Autodesk Inventor part; units mm, degrees
ref_plane "YZ Plane" through (0, 0, 0) normal (1, 0, 0) x (0, 1, 0)
ref_plane "XZ Plane" through (0, 0, 0) normal (0, 1, 0) x (-1, 0, 0)
ref_plane "XY Plane" through (0, 0, 0) normal (0, 0, 1) x (1, 0, 0)
sketch "Sketch1" plane through (0, 0, 0) normal (0, 1, 0) x (-1, 0, 0)
  line L0 (-152.4, 28.575) -> (152.4, 28.575)
  line L1 (152.4, 28.575) -> (152.4, -28.575)
  line L2 (152.4, -28.575) -> (-152.4, -28.575)
  line L3 (-152.4, -28.575) -> (-152.4, 28.575)
  line L4 (-152.4, 28.575) -> (152.4, -28.575) construction
  line L5 (152.4, 28.575) -> (-152.4, -28.575) construction
  point P0 (0, 0)
  dimension "d0" = 304.8
  dimension "d1" = 57.15
extrude "Extrusion1" add sketch "Sketch1" along normal blind 3.175
sketch "Sketch2" plane through (0, 3.175, 0) normal (0, 1, 0) x (1, 0, 0)
  line L0 (152.4, 28.575) -> (-152.4, 28.575)
  line L1 (-152.4, -28.575) -> (152.4, -28.575)
  line L2 (0, -15.875) -> (-152.4, -15.875)
  line L3 (-152.4, 28.575) -> (-152.4, -28.575)
  line L4 (0, -15.875) -> (152.4, -15.875)
  line L5 (0, 15.875) -> (-152.4, 15.875)
  line L6 (0, 15.875) -> (152.4, 15.875)
  line L7 (152.4, -28.575) -> (152.4, 28.575)
  line L8 (-152.4, -15.875) -> (-107.95, -15.875)
  line L9 (-107.95, -15.875) -> (-63.5, -15.875)
  line L10 (-63.5, -15.875) -> (-19.05, -15.875)
  line L11 (-19.05, -15.875) -> (25.4, -15.875)
  line L12 (25.4, -15.875) -> (69.85, -15.875)
  line L13 (69.85, -15.875) -> (114.3, -15.875)
  line L14 (-152.4, 15.875) -> (-127, 15.875)
  line L15 (-127, 15.875) -> (-50.8, 15.875)
  line L16 (-50.8, 15.875) -> (25.4, 15.875)
  line L17 (25.4, 15.875) -> (101.6, 15.875)
  point P0 (0, 0)
  dimension "d8" = 44.45
  dimension "d9" = 44.45
  dimension "d10" = 44.45
  dimension "d11" = 44.45
  dimension "d12" = 44.45
  dimension "d13" = 44.45
  dimension "d14" = 25.4
  dimension "d15" = 76.2
  dimension "d16" = 76.2
  dimension "d17" = 76.2
hole "Hole1" at (-107.95, 3.175, 15.875) at (-63.5, 3.175, 15.875) at (-19.05, 3.175, 15.875) at (25.4, 3.175, 15.875) at (69.85, 3.175, 15.875) at (114.3, 3.175, 15.875) direction (0, -1, 0) diameter 5.1054 end through all
sketch "Sketch3" plane through (0, 3.175, 0) normal (0, 1, 0) x (1, 0, 0)
  line L0 (152.4, 28.575) -> (-152.4, 28.575)
  line L1 (-152.4, -28.575) -> (152.4, -28.575)
  line L2 (0, -15.875) -> (-152.4, -15.875)
  line L3 (-152.4, 28.575) -> (-152.4, -28.575)
  line L4 (0, -15.875) -> (152.4, -15.875)
  line L5 (0, 15.875) -> (-152.4, 15.875)
  line L6 (0, 15.875) -> (152.4, 15.875)
  line L7 (152.4, -28.575) -> (152.4, 28.575)
  line L8 (-152.4, -15.875) -> (-107.95, -15.875)
  line L9 (-107.95, -15.875) -> (-63.5, -15.875)
  line L10 (-63.5, -15.875) -> (-19.05, -15.875)
  line L11 (-19.05, -15.875) -> (25.4, -15.875)
  line L12 (25.4, -15.875) -> (69.85, -15.875)
  line L13 (69.85, -15.875) -> (114.3, -15.875)
  line L14 (-152.4, 15.875) -> (-127, 15.875)
  line L15 (-127, 15.875) -> (-50.8, 15.875)
  line L16 (-50.8, 15.875) -> (25.4, 15.875)
  line L17 (25.4, 15.875) -> (101.6, 15.875)
  point P0 (0, 0)
  point P1 (0, 0)
  dimension "d25" = 44.45
  dimension "d26" = 44.45
  dimension "d27" = 44.45
  dimension "d28" = 44.45
  dimension "d29" = 44.45
  dimension "d30" = 44.45
  dimension "d31" = 25.4
  dimension "d32" = 76.2
  dimension "d33" = 76.2
  dimension "d34" = 76.2
hole "Hole2" at (-127, 3.175, -15.875) at (-50.8, 3.175, -15.875) at (25.4, 3.175, -15.875) at (101.6, 3.175, -15.875) direction (0, -1, 0) diameter 3.81 end through all
properties part number "Rack-Elondo-Bracket"
Check sheet for the modelled part. Datum: model origin and axes. Units: mm. Round coordinates to 2 decimals unless told otherwise and drop trailing zeros. Loops run counter-clockwise (first coordinate to the right, second up) from the corner with the lowest first, then second, coordinate; pieces in that order, holes last. Notation, with made-up numbers: (18.25, -20) - (72.25, -20) arc R30 cw to (72.25, 18) - close; hole circle Ø8 at (20, 6.25). An arc over 180 degrees is marked (long way). Write item = value, one per line. Start each with the question number.
Q1. Release check for a two-part mould opening along Z. For faces 1 (the face through (2, 0, 0)), 2 (the face through (67.32, 1.57, 15.54)) record: pulls with the +Z half, pulls with the -Z half, needs draft (parallel to the pull), parting line crosses it, or undercut.
Q2. Thickness scan on L1, parallel to Z at x = 25.4, y = 2 (3 decimals); L2, parallel to Z at x = -19.05, y = 2.4 (3 decimals); L3, parallel to Z at x = 101.6, y = 1.3 (3 decimals). Record the ranges inside material, lowest first.
Q3. Section check A-A (x = -19.05). Record the boundary of the cut face in (y, z) (3 decimals).
Derived:
q1.face_1 = needs draft
q1.face_2 = undercut
q2.L1 = -28.575 to -17.78, -13.97 to 13.322, 18.428 to 28.575
q2.L2 = -28.575 to 13.322, 18.428 to 28.575
q2.L3 = -28.575 to -17.78, -13.97 to 28.575
q3.outline = (0, -28.575) - (3.175, -28.575) - (3.175, 13.322) - (0, 13.322) - close; (0, 18.428) - (3.175, 18.428) - (3.175, 28.575) - (0, 28.575) - close
